```python
from build123d import *

# Parameters (mm, degrees)
SKETCH1_W           = 61
SKETCH1_H           = 6.1
BOSS_EXTRUDE1_DEPTH = 22.5
SKETCH2_OUTSIDE_W   = 76.06
SKETCH2_OUTSIDE_H   = 21.16
SKETCH2_OUTSIDE_W_2 = 61
SKETCH2_OUTSIDE_H_2 = 5.41284
CUT_EXTRUDE1_DEPTH  = 6
CUT_EXTRUDE3_DEPTH  = 23.5
SKETCH6_R           = 3.175
CUT_EXTRUDE4_DEPTH  = 7.1
SKETCH7_R           = 1.5
CUT_EXTRUDE5_DEPTH  = 7.1


with BuildPart() as part:
    # Sketch1 → Boss-Extrude1 (new body)
    with BuildSketch(Plane(origin=(0, 0, 0), x_dir=(0, 0, -1), z_dir=(1, 0, 0))):
        with Locations((30.5, 0)):
            Rectangle(SKETCH1_W, SKETCH1_H)
    extrude(amount=BOSS_EXTRUDE1_DEPTH)

    # Sketch2 outside → Cut-Extrude1 (cut)
    with BuildSketch(Plane(origin=(22.5, 0, 0), x_dir=(0, 0, -1), z_dir=(1, 0, 0))):
        with Locations((30.5, 0)):
            Rectangle(SKETCH2_OUTSIDE_W, SKETCH2_OUTSIDE_H)
        with Locations((30.5, 0)):
            Rectangle(SKETCH2_OUTSIDE_W_2, SKETCH2_OUTSIDE_H_2, mode=Mode.SUBTRACT)
    extrude(amount=-CUT_EXTRUDE1_DEPTH, mode=Mode.SUBTRACT)

    # Sketch5 → Cut-Extrude3 (cut, through all)
    with BuildSketch(Plane.ZY):
        with BuildLine():
            Line((-43.5866, -0.01898), (-43.5866, -3.05))
            Line((-43.5866, -3.05), (-48.6514, -3.05))
            Line((-48.6514, -3.05), (-48.6514, -0.01898))
            ThreePointArc((-48.6514, -0.01898), (-46.119, 2.51342), (-43.5866, -0.01898))
        make_face()
    extrude(amount=-CUT_EXTRUDE3_DEPTH, mode=Mode.SUBTRACT)

    # Sketch6 → Cut-Extrude4 (cut, through all)
    with BuildSketch(Plane(origin=(0, 3.05, 0), x_dir=(1, 0, 0), z_dir=(0, 1, 0))):
        with Locations(Location((7.5, 30.5, 0), (0, 0, 270))):  # turned: the seam where the file's is
            Circle(SKETCH6_R)
    extrude(amount=-CUT_EXTRUDE4_DEPTH, mode=Mode.SUBTRACT)

    # Sketch7 → Cut-Extrude5 (cut, through all)
    with BuildSketch(Plane(origin=(0, 3.05, 0), x_dir=(1, 0, 0), z_dir=(0, 1, 0))):
        with Locations(Location((5, 55.5, 0), (0, 0, 270))):  # turned: the seam where the file's is
            Circle(SKETCH7_R)
        with Locations(Location((5, 5.5, 0), (0, 0, 270))):  # turned: the seam where the file's is
            Circle(SKETCH7_R)
    extrude(amount=-CUT_EXTRUDE5_DEPTH, mode=Mode.SUBTRACT)


solid = part.part
```
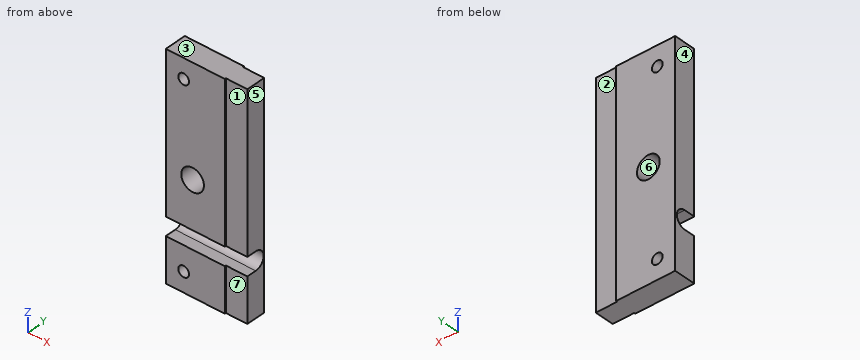
Work out the finished part from the listing and answer in its coordinate system (mm). Face numbers are marked on the shaded views. A direction names the side the tool comes from. Round coordinates to 2 decimals unless told otherwise and drop trailing zeros. Write each loop counter-clockwise with the first axis right and the second up, starting at its lowest first coordinate (ties: lowest second). Pieces come first, ordered by that corner, then holes. Notation, with made-up numbers: (69.5, 32.5) -> (106.5, 32.5) arc R15 ccw to (106.5, 57.5) -> close; hole circle Ø4 at (41.25, 52). An arc over 180 degrees is marked (long way). Write each question's results on one line, items separated by ' | '.
Q1. Section A-A, the plane x = 7.5 is taken. Write down the section's boundary in (y, z) (3 decimals), then the cut area to 3 significant figures.
Data:
outline: (-3.05, -61) -> (3.05, -61) -> (3.05, -33.675) -> (-3.05, -33.675) -> (-3.05, -43.587) -> (-0.019, -43.587) arc R2.532 cw to (-0.019, -48.651) -> (-3.05, -48.651) -> close; (-3.05, -27.325) -> (3.05, -27.325) -> (3.05, 0) -> (-3.05, 0) -> close | area: 308 mm^2
Q2. Determine the mould class of the marked faces 4, 5, 6 and 7 for opening direction X: released by +X, released by -X, zero draft, split by the parting line, or undercut.
Data:
face 4: released by -X | face 5: released by +X | face 6: undercut | face 7: zero draft
Q3. Section B-B, the plane z = -30.5 is taken. Write down the section's boundary in (x, y) (3 decimals).
Data:
outline: (0, -3.05) -> (4.325, -3.05) -> (4.325, 3.05) -> (0, 3.05) -> close; (10.675, -3.05) -> (16.5, -3.05) -> (16.5, -2.706) -> (22.5, -2.706) -> (22.5, 2.706) -> (16.5, 2.706) -> (16.5, 3.05) -> (10.675, 3.05) -> close
Q4. Straight lines are drawn through the part: line 1 along X through (y, z) = (-0.5, -30.5) (3 decimals); line 2 along Z through (x, y) = (3, 0); line 3 along X through (y, z) = (-0.25, -55.5). For each, find the intervals that lie inside material, in ascending order. Write a range as [from, to].
Data:
line 1: [0, 4.325], [10.675, 22.5] | line 2: [-61, -48.65], [-43.59, 0] | line 3: [0, 3.5], [6.5, 22.5]
Q5. Section D-D, the plane x = 17.25 is taken. Write down the section's boundary in (y, z), then the cut area to 3 significant figures.
Data:
outline: (-2.71, -61) -> (2.71, -61) -> (2.71, 0) -> (-2.71, 0) -> (-2.71, -43.59) -> (-0.02, -43.59) arc R2.53 cw to (-0.02, -48.65) -> (-2.71, -48.65) -> close | area: 306 mm^2
Q6. Which of the six approach directions +Z, -Z, +X, -X, +Y, -Y give full straight-line access (tool end or side, diameter ignored) to the marked faces 1, 2 and 3?
Data:
face 1: +Z, -Z, +X, -Y | face 2: +Z, -Z, +X, +Y | face 3: +Z, +X, -X, +Y, -Y
Q7. Section C-C, the plane y = -1.25 is taken. Write down the section's boundary in (x, z) (3 decimals).
Data:
outline: (0, -61) -> (22.5, -61) -> (22.5, -48.651) -> (0, -48.651) -> close; (0, -43.587) -> (22.5, -43.587) -> (22.5, 0) -> (0, 0) -> close; hole circle Ø3 at (5, -55.5); hole circle Ø3 at (5, -5.5); hole circle Ø6.35 at (7.5, -30.5)
